Geometry: final body of the model. Coordinates: model frame, mm. Round coordinates to 2 decimals unless told otherwise and drop trailing zeros. Loops run counter-clockwise (first coordinate to the right, second up) from the corner with the lowest first, then second, coordinate; pieces in that order, holes last. Notation, with made-up numbers: (25, 20) - (54, 20) arc R7 cw to (54, 27) - close; hole circle Ø7 at (22, 67). An arc over 180 degrees is marked (long way). Write item = value, one per line. Start each with the question number.
Item 1: Section B-B (z = 233.5). Return loops of the section in (x, y) (3 decimals), plus the area to 3 significant figures.
Item 2: Section A-A (y = 0.85). Return loops of the section in (x, z) (3 decimals), plus the area to 3 significant figures.
Item 3: First-contact query: pin 1 (1 mm diameter, centred on y = 1.5, z = 28, fed in from -X); pin 2 (1.6 mm diameter, centred on x = 252, y = 1, fed in from +Z); pin 3 (1 mm diameter, centred on x = 251.5, y = 1.5, fed in from -Z). Flat tips, straight axial feed; report the tip coordinate or a pass-through.
Item 4: Line query: line 1 (X direction, y = 1.5, z = 120). Output: solid intervals per line, ascending. Write a range as from..to.
from build123d import *

# Parameters (mm, degrees)
SKETCH1_W           = 250
SKETCH1_H           = 320
BOSS_EXTRUDE1_DEPTH = 3.175
SKETCH2_W           = 3.175
SKETCH2_H           = 40
BOSS_EXTRUDE2_DEPTH = 3.175


with BuildPart() as part:
    # Sketch1 → Boss-Extrude1 (new body)
    with BuildSketch(Plane(origin=(0, 0, 0), x_dir=(1, 0, 0), z_dir=(0, 1, 0))):
        with Locations((125, -160)):
            Rectangle(SKETCH1_W, SKETCH1_H)
    extrude(amount=BOSS_EXTRUDE1_DEPTH)

    # Sketch2 → Boss-Extrude2 (add)
    with BuildSketch(Plane(origin=(0, 3.175, 0), x_dir=(1, 0, 0), z_dir=(0, 1, 0))):
        with Locations((-1.5875, -60)):
            Rectangle(SKETCH2_W, SKETCH2_H)
        with Locations((251.5875, -60)):
            Rectangle(SKETCH2_W, SKETCH2_H)
        with Locations((251.5875, -160)):
            Rectangle(SKETCH2_W, SKETCH2_H)
        with Locations((-1.5875, -160)):
            Rectangle(SKETCH2_W, SKETCH2_H)
        with Locations((251.5875, -260)):
            Rectangle(SKETCH2_W, SKETCH2_H)
        with Locations((-1.5875, -260)):
            Rectangle(SKETCH2_W, SKETCH2_H)
    extrude(amount=-BOSS_EXTRUDE2_DEPTH)


solid = part.part
Taken from the geometry:
q1.outline = (0, 0) - (250, 0) - (250, 3.175) - (0, 3.175) - close
q1.area = 794 mm^2
q2.outline = (-3.175, 40) - (0, 40) - (0, 0) - (250, 0) - (250, 40) - (253.175, 40) - (253.175, 80) - (250, 80) - (250, 140) - (253.175, 140) - (253.175, 180) - (250, 180) - (250, 240) - (253.175, 240) - (253.175, 280) - (250, 280) - (250, 320) - (0, 320) - (0, 280) - (-3.175, 280) - (-3.175, 240) - (0, 240) - (0, 180) - (-3.175, 180) - (-3.175, 140) - (0, 140) - (0, 80) - (-3.175, 80) - close
q2.area = 80,800 mm^2
q3.pin_1 = 0
q3.pin_2 = 280
q3.pin_3 = 40
q4.line_1 = 0..250
